Geometry check sheet. Reference: the model listing, model coordinates, mm. Round coordinates to 2 decimals unless told otherwise and drop trailing zeros. Loops run counter-clockwise (first coordinate to the right, second up) from the corner with the lowest first, then second, coordinate; pieces in that order, holes last. Notation, with made-up numbers: M 62,-25.75 L 116,-25.75 A15 ccw 116,-14.75 Z; hole C 47,-38.75 d2. An arc over 180 degrees is marked long. Write item = value, one per line.
from build123d import *

# Parameters (mm, degrees)
SKETCH_1_W = 494
SKETCH_1_H = 10


with BuildPart() as part:
    # 草图1 → 旋转1 (revolve)
    with BuildSketch(Plane.XY):
        Polygon((-265, 0), (-265, 10), (-253, 10), (-253, 12), (-250, 12), (-250, 25), (250, 25), (250, 12), (253, 12), (253, 10), (265, 10), (265, 0), align=None)
        with Locations((0, 17)):
            Rectangle(SKETCH_1_W, SKETCH_1_H, mode=Mode.SUBTRACT)
    revolve(axis=Axis((265, 0, 0), (-1, 0, 0)))


solid = part.part
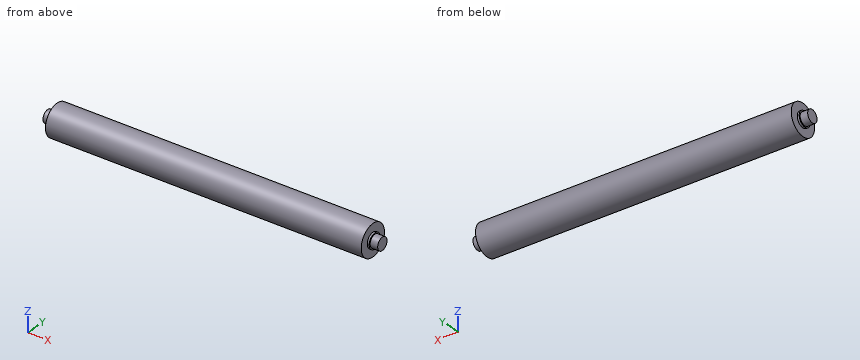
(1) Material ranges on line 1 along Z through (x, y) = (-5, 0); line 2 along X through (y, z) = (-15, 2.5), recorded low to high. Write a range as from..to.
Result set:
line_1 = -25..-22, -12..12, 22..25
line_2 = -250..-247, 247..250
(2) Depth check by flat-ended pin: pin 1 Ø5 at (y, z) = (13.5, -3.5) entering from -X; pin 2 Ø6 at (x, y) = (19, 17.5) entering from -Z; pin 3 Ø1.5 at (x, y) = (-135.5, 1) entering from -Z. Enter the tip coordinate at first touch or a pass-through.
Result set:
pin_1 = -253
pin_2 = -20.37
pin_3 = -25
(3) Sectioned sample at C-C on x = -100.5. Record the cut outline in (y, z), then the cut area to 3 significant figures.
Result set:
outline = C 0,0 d50; C 0,0 d24; hole C 0,0 d44
area = 895 mm2
(4) Sectioned sample at A-A on y = 0. Record the cut outline in (x, z), then the cut area to 3 significant figures.
Result set:
outline = M -265,-10 L -253,-10 L -253,-12 L -250,-12 L -250,-25 L 250,-25 L 250,-12 L 253,-12 L 253,-10 L 265,-10 L 265,10 L 253,10 L 253,12 L 250,12 L 250,25 L -250,25 L -250,12 L -253,12 L -253,10 L -265,10 Z; hole M -247,-22 L 247,-22 L 247,-12 L -247,-12 Z; hole M -247,12 L 247,12 L 247,22 L -247,22 Z
area = 15,700 mm2
